from build123d import *

# Parameters (mm, degrees)
F0_W     = 36.04
F0_H     = 23.04
F1_DEPTH = 7.74
F2_W     = 25.98
F2_H     = 23.04
F3_DEPTH = 4.88
F4_R     = 6.55
F5_DEPTH = 12.621
F6_SIZE2 = 0.175
F6_SIZE  = 0.175


with BuildPart() as f1:
    # F0 (on Top) → F1 (new body)
    with BuildSketch(Plane.XY):
        with Locations((18.02, 11.52)):
            Rectangle(F0_W, F0_H)
    extrude(amount=F1_DEPTH)

    # F2 (on face) → F3 (join)
    with BuildSketch(Plane.XY.offset(7.74)):
        with Locations((12.99, 11.52)):
            Rectangle(F2_W, F2_H)
    extrude(amount=F3_DEPTH)

    # F4 (on face) → F5 (cut, through all)
    with BuildSketch(Plane.XY.offset(12.62)):
        with Locations((13.93, 11.65)):
            Circle(F4_R)
    extrude(amount=-F5_DEPTH, mode=Mode.SUBTRACT)

    # F6
    f6_edges = [f1.edges().sort_by_distance(p)[0] for p in [
        (7.38, 11.65, 12.62),
        (7.38, 11.65, 0),
    ]]
    chamfer(f6_edges, length=F6_SIZE, length2=F6_SIZE2)


solid = f1.part
Verification items for the finished model (mm, model axes). A direction names the side the tool comes from. Coordinates: 2 decimals unless noted, no trailing zeros. Write each loop counter-clockwise with the first axis right and the second up, starting at its lowest first coordinate (ties: lowest second). Pieces come first, ordered by that corner, then holes. Notation, with made-up numbers: (51.5, -12.5) -> (73.5, -12.5) arc R8 ccw to (73.5, -4.5) -> close; hole circle Ø5 at (-38, -1.5). An arc over 180 degrees is marked (long way). One line per item, written item: value. Start each with the question number.
Q1. Access from +Z, -Z, +X, -X, +Y, -Y to the whole of each face (thin tool, end or side, straight path). Record for faces 5 (the flat face through (7, 12, 12.62)), 6 (the flat face through (25.98, 11, 10)).
Q2. Cross-section at D-D on x = 30. Enter the section's corners in (y, z), and give its area (3 significant figures).
Q3. Go/stop test with flat-tipped pins: P1, Ø4, axis at y = 13.5, z = 10, coming from the +X side; P2, Ø8, axis at x = 31, y = 9.5, coming from the +Z side. Record where each tip stops, or that it passes through.
Q4. Cross-section at C-C on z = 1.5. Enter the section's corners in (x, y).
Q5. Mould release check, pull along Y, two halves, no side actions. Record for faces 1 (the flat face through (18, 0, 6)), 2 (the cylindrical face through (8.732, 7.664, 6.396)), 3 (the flat face through (18, 23.04, 6)), 4 (the flat face through (31, 12, 7.74)): pulls with the +Y half, pulls with the -Y half, needs draft (parallel to the pull), parting line crosses it, or undercut.
Q6. Cross-section at B-B on x = 13.93. Enter the section's corners in (y, z) (3 decimals).
Q7. Cross-section at A-A on y = 11.65. Enter the section's corners in (x, z) (3 decimals), and give its area (3 significant figures).
Q8. Thickness scan on L1, parallel to Y at x = 13.93, z = 4.75; L2, parallel to Y at x = 16, z = 9.25; L3, parallel to Z at x = 31, y = 1.75. Record the ranges inside material, lowest first. Write a range as from..to.
Checked values:
1. face 5: +Z, +X, -X, +Y, -Y
1. face 6: +Z, +X, +Y, -Y
2. outline: (0, 0) -> (23.04, 0) -> (23.04, 7.74) -> (0, 7.74) -> close
2. area: 178 mm²
3. P1: stops at x = 25.98
3. P2: stops at z = 7.74
4. outline: (0, 0) -> (36.04, 0) -> (36.04, 23.04) -> (0, 23.04) -> close; hole circle Ø13.1 at (13.93, 11.65)
5. face 1: pulls with the -Y half
5. face 2: undercut
5. face 3: pulls with the +Y half
5. face 4: needs draft
6. outline: (0, 0) -> (4.925, 0) -> (5.1, 0.175) -> (5.1, 12.445) -> (4.925, 12.62) -> (0, 12.62) -> close; (18.2, 0.175) -> (18.375, 0) -> (23.04, 0) -> (23.04, 12.62) -> (18.375, 12.62) -> (18.2, 12.445) -> close
7. outline: (0, 0) -> (7.205, 0) -> (7.38, 0.175) -> (7.38, 12.445) -> (7.205, 12.62) -> (0, 12.62) -> close; (20.48, 0.175) -> (20.655, 0) -> (36.04, 0) -> (36.04, 7.74) -> (25.98, 7.74) -> (25.98, 12.62) -> (20.655, 12.62) -> (20.48, 12.445) -> close
7. area: 240 mm²
8. L1: y = 0..5.1, 18.2..23.04
8. L2: y = 0..5.44, 17.86..23.04
8. L3: z = 0..7.74
